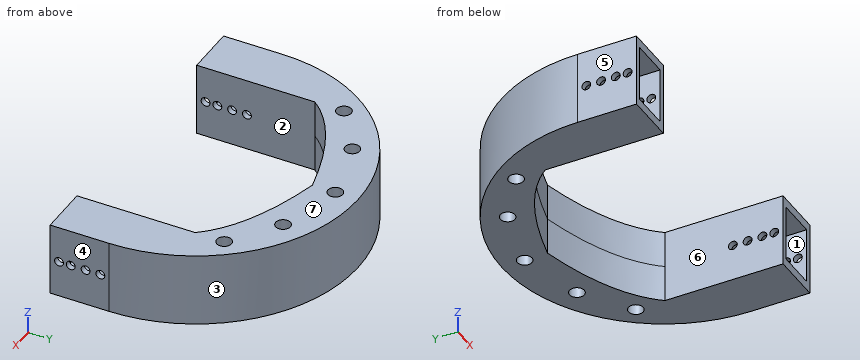
```python
from build123d import *

# Parameters (mm, degrees)
BOSS_EXTRUDE2_DEPTH = 12.5
SKETCH2_W           = 17
SKETCH2_H           = 25
BOSS_EXTRUDE3_DEPTH = 20
SKETCH3_W           = 13
SKETCH3_H           = 19
CUT_EXTRUDE1_DEPTH  = 30
SKETCH4_R           = 1.5
CUT_EXTRUDE2_DEPTH  = 124.617353294
SKETCH5_R           = 2.5
CUT_EXTRUDE3_DEPTH  = 30


with BuildPart() as part:
    # Sketch1 → Boss-Extrude2 (new, symmetric)
    with BuildSketch(Plane.XY):
        with BuildLine():
            Line((-55, 0), (-38, 0))
            Line((-38, 0), (-38, 20))
            add(Edge.make_bspline(
                [(0, 39.5), (-28.167603026, 32.926551341), (-38, 20)],
                knots=[0, 0, 0, 0.331450034, 0.331450034, 0.331450034], degree=2))
            add(Edge.make_bspline(
                [(0, 39.5), (28.167603026, 32.926551341), (38, 20)],
                knots=[0, 0, 0, 0.331450034, 0.331450034, 0.331450034], degree=2))
            Line((38, 20), (38, 0))
            Line((38, 0), (55, 0))
            ThreePointArc((55, 0), (0, 55), (-55, 0))
        make_face()
    extrude(amount=BOSS_EXTRUDE2_DEPTH, both=True)

    # Sketch2 → Boss-Extrude3 (add)
    with BuildSketch(Plane.XZ):
        with Locations((46.5, 0)):
            Rectangle(SKETCH2_W, SKETCH2_H)
        with Locations((-46.5, 0)):
            Rectangle(SKETCH2_W, SKETCH2_H)
    extrude(amount=BOSS_EXTRUDE3_DEPTH)

    # Sketch3 → Cut-Extrude1 (cut)
    with BuildSketch(Plane.XZ.offset(20)):
        with Locations((-46.5, 0)):
            Rectangle(SKETCH3_W, SKETCH3_H)
        with Locations((46.5, 0)):
            Rectangle(SKETCH3_W, SKETCH3_H)
    extrude(amount=-CUT_EXTRUDE1_DEPTH, mode=Mode.SUBTRACT)

    # Sketch4 → Cut-Extrude2 (cut, through all)
    with BuildSketch(Plane.ZY.offset(55)):
        with Locations((0, -3)):
            Circle(SKETCH4_R)
        with Locations((0, -17)):
            Circle(SKETCH4_R)
        with Locations((0, -8)):
            Circle(SKETCH4_R)
        with Locations((0, -13)):
            Circle(SKETCH4_R)
    extrude(amount=-CUT_EXTRUDE2_DEPTH, mode=Mode.SUBTRACT)

    # Sketch5 → Cut-Extrude3 (cut)
    with BuildSketch(Plane.XY.offset(12.5)):
        with Locations((0, 47.25)):
            Circle(SKETCH5_R)
        with Locations((-38, 29.880895352)):
            Circle(SKETCH5_R)
        with Locations((38, 29.880895352)):
            Circle(SKETCH5_R)
        with Locations((-22, 41.266508356)):
            Circle(SKETCH5_R)
        with Locations((22, 41.266508356)):
            Circle(SKETCH5_R)
    extrude(amount=-CUT_EXTRUDE3_DEPTH, mode=Mode.SUBTRACT)


solid = part.part
```
Check sheet for the modelled part. Datum: model origin and axes. Units: mm. Face numbers are marked on the shaded views. A direction names the side the tool comes from. Coordinates: 2 decimals unless noted, no trailing zeros. Loops run counter-clockwise (first coordinate to the right, second up) from the corner with the lowest first, then second, coordinate; pieces in that order, holes last.
1) Sectioned sample at A-A (y = -3). Count the separate pieces of the cut face and the enclosed holes in it, and give its area (3 significant figures).
2) Gauge pin test, flat ends, axial feed: pin 1 (12 mm diameter, centred on y = 9, z = 3, fed in from +X); pin 2 (8 mm diameter, centred on y = 23, z = -3, fed in from -X); pin 3 (8 mm diameter, centred on x = 29, z = -7.5, fed in from +Y); pin 4 (8 mm diameter, centred on x = 0, y = 47.25, fed in from +Z). Record the tip position at first contact, or that the pin passes through.
3) Access from +Z, -Z, +X, -X, +Y, -Y to the whole of each face (thin tool, end or side, straight path). Record for the marked faces 1, 2 and 3.
4) Sectioned sample at B-B (y = 47.25). Record the boundary of the cut face in (x, z).
5) Material ranges on probe 1 along X at (y, z) = (-3, 8.25); probe 2 along Z at (x, y) = (-45, -14.5); probe 3 along Y at (x, z) = (38.8, 0), recorded low to high.
6) Release check for a two-part mould opening along X. For the marked faces 4, 5, 6 and 7 record: released by +X, released by -X, zero draft, split by the parting line, or undercut.
Check sheet entries:
1. separate pieces: 4
1. enclosed holes: 0
1. area: 332 mm2
2. pin 1: stops at x = 54.92
2. pin 2: stops at x = -51.61
2. pin 3: stops at y = 48.99
2. pin 4: stops at z = 12.5
3. face 1: -Y
3. face 2: +Z, -Z, -Y
3. face 3: +Z, -Z, +Y
4. outline: (-28.15, -12.5) - (-2.5, -12.5) - (-2.5, 12.5) - (-28.15, 12.5) - close; (2.5, -12.5) - (28.15, -12.5) - (28.15, 12.5) - (2.5, 12.5) - close
5. probe 1: x = -55 to -53, -40 to -38, 38 to 40, 53 to 55
5. probe 2: z = -12.5 to -9.5, 9.5 to 12.5
5. probe 3: y = -20 to -18.5, -15.5 to -14.5, -11.5 to -9.5, -6.5 to -4.5, -1.5 to 27.51, 32.25 to 38.98
6. face 4: released by +X
6. face 5: released by -X
6. face 6: undercut
6. face 7: zero draft
